```python
from build123d import *

# Parameters (mm, degrees)
SKETCH_1_W          = 30
SKETCH_1_H          = 10
SKETCH_1_W_2        = 26
SKETCH_1_H_2        = 6
EXTRUDE_1_DEPTH     = 330
SKETCH_2_R          = 1.6
CUT_EXTRUDE_1_DEPTH = 331.492057393
SKETCH_3_R          = 1.6
SKETCH_3_R_2        = 1.65
CUT_EXTRUDE_2_DEPTH = 331.492057393
SKETCH_4_R          = 1.6
CUT_EXTRUDE_3_DEPTH = 332.398551596


with BuildPart() as part:
    # 草图1 → 凸台-拉伸1 (new body)
    with BuildSketch(Plane.XY):
        Rectangle(SKETCH_1_W, SKETCH_1_H)
        Rectangle(SKETCH_1_W_2, SKETCH_1_H_2, mode=Mode.SUBTRACT)
    extrude(amount=EXTRUDE_1_DEPTH)

    # 草图2 → 切除-拉伸1 (cut, through all)
    with BuildSketch(Plane(origin=(0, 5, 0), x_dir=(1, 0, 0), z_dir=(0, 1, 0))):
        with Locations(Location((-11.3, -321, 0), (0, 0, 270))):
            Circle(SKETCH_2_R)
    extrude(amount=-CUT_EXTRUDE_1_DEPTH, mode=Mode.SUBTRACT)

    # 草图3 → 切除-拉伸2 (cut, through all)
    with BuildSketch(Plane(origin=(0, 5, 0), x_dir=(1, 0, 0), z_dir=(0, 1, 0))):
        with Locations(Location((5.907293091, -296.425438671, 0), (0, 0, 270))):
            Circle(SKETCH_3_R)
        with Locations(Location((0, -163.912345182, 0), (0, 0, 270))):
            Circle(SKETCH_3_R_2)
        with Locations(Location((0, -133.912345182, 0), (0, 0, 270))):
            Circle(SKETCH_3_R_2)
        with Locations(Location((0, -223.912345182, 0), (0, 0, 270))):
            Circle(SKETCH_3_R_2)
        with Locations(Location((0, -193.912345182, 0), (0, 0, 270))):
            Circle(SKETCH_3_R_2)
    extrude(amount=-CUT_EXTRUDE_2_DEPTH, mode=Mode.SUBTRACT)

    # 草图4 → 切除-拉伸3 (cut, through all)
    with BuildSketch(Plane.ZY.offset(15)):
        with Locations((20, 0)):
            Circle(SKETCH_4_R)
        with Locations((40, 0)):
            Circle(SKETCH_4_R)
        with Locations((60, 0)):
            Circle(SKETCH_4_R)
    extrude(amount=-CUT_EXTRUDE_3_DEPTH, mode=Mode.SUBTRACT)


solid = part.part
```
Can you work these out from the model? Positions are in its coordinate system, mm. A direction names the side the tool comes from. Give positions to 0.01 mm unless a question says otherwise; leave off trailing zeros. Loops run counter-clockwise (first coordinate to the right, second up) from the corner with the lowest first, then second, coordinate; pieces in that order, holes last. Notation, with made-up numbers: M -14.75,74 L -3.75,74 A23 ccw -3.75,86 Z; hole C 79,0.25 d4. An arc over 180 degrees is marked long. One line per item, written item: value.
(1) I need wall thicknesses on line 1 (Y direction, x = 10.5, z = 279.5); line 2 (X direction, y = -3.75, z = 321); line 3 (X direction, y = -1, z = 99.5). Which ranges of each line are inside material? Lowest first, please.
Returned:
line 1: -5 to -3, 3 to 5
line 2: -15 to -12.9, -9.7 to 15
line 3: -15 to -13, 13 to 15
(2) Suppose I cut it at C-C on y = 0. Count the separate pieces of the cut face and the enclosed holes in it, plus the area to 3 significant figures.
Returned:
separate pieces: 8
enclosed holes: 0
area: 1,280 mm^2
(3) Suppose I cut it at A-A on z = 180. List the corners of the cut face in (x, y) for me, plus the area to 3 significant figures.
Returned:
outline: M -15,-5 L 15,-5 L 15,5 L -15,5 Z; hole M -13,-3 L 13,-3 L 13,3 L -13,3 Z
area: 144 mm^2
(4) We'd pull the mould along X, two halves only. Please class faces 3 (the face through (15, 0, 163)), 4 (the face through (-13, 0, 163)), 5 (the face through (-0.2, 3.4, 330)): released by +X, released by -X, zero draft, split by the parting line, or undercut.
Returned:
face 3: released by +X
face 4: undercut
face 5: zero draft
(5) Suppose I cut it at B-B on x = -6.5. List the corners of the cut face in (y, z) for me.
Returned:
outline: M -5,0 L -3,0 L -3,330 L -5,330 Z; M 3,0 L 5,0 L 5,330 L 3,330 Z
(6) Which directions (+Z, -Z, +X, -X, +Y, -Y) give clear straight access to the entire face, cutting with the end or side of a thin tool? Please do faces 1 (the face through (-4, 5, 163)), 2 (the face through (13, 0, 163)).
Returned:
face 1: +Z, -Z, +X, -X, +Y
face 2: +Z, -Z
